Read the model definition and answer for the solid it produces. Units are mm, in the model's axes. Face numbers are marked on the shaded views. A direction names the side the tool comes from. Round coordinates to 2 decimals unless told otherwise and drop trailing zeros. Order: outer loops, then holes, each group sorted by start corner. A loop starts at its lowest first (then second) coordinate and runs counter-clockwise, first axis right, second up. Notation, with made-up numbers: (81.5, 11.25) -> (97.5, 11.25) arc R9 ccw to (97.5, 26.25) -> close; hole circle Ø2 at (59, 86). An arc over 180 degrees is marked (long way). One line per item, written item: value. Start each with the question number.
1. Flat-ended cylindrical pins translate along their axes: pin 1 Ø2.5 at (y, z) = (1.5, -3) entering from +X; pin 2 Ø4 at (x, y) = (34, 6.5) entering from +Z. Find the tip coordinate at first contact, or state that the pin passes through.
2. Section A-A (x = 32) is taken. Give the vertices of the cut face in (y, z), then the cut area to 3 significant figures.
3. The mould has two halves that part along Z. Classify the marked faces 3, 4 and 5: released by +Z, released by -Z, zero draft, split by the parting line, or undercut.
4. Section C-C (z = -2) is taken. Give the vertices of the cut face in (x, y).
5. Section D-D (x = 16.5) is taken. Give the vertices of the cut face in (y, z).
6. For the marked faces 1 and 2, determine the directions among +Z, -Z, +X, -X, +Y, -Y from which every point of the face is accessible in a straight line to the end or side of a thin tool.
7. Consider line 1 (Z direction, x = 25, y = 6); line 2 (X direction, y = 2, z = -2.5); line 3 (X direction, y = 5.75, z = -4.25). Determine where each line is inside the solid, lowest interval first.
8. Section B-B (y = 1.5) is taken. Give the vertices of the cut face in (x, z), then the cut area to 3 significant figures.
from build123d import *

# Parameters (mm, degrees)
SKETCH1_W           = 6.35
SKETCH1_H           = 12.192
BOSS_EXTRUDE1_DEPTH = 25.4
SKETCH2_W           = 1.6002
SKETCH2_H           = 12.192
BOSS_EXTRUDE2_DEPTH = 12.7
CHAMFER1_SIZE       = 10


with BuildPart() as part:
    # Sketch1 → Boss-Extrude1 (new body)
    with BuildSketch(Plane(origin=(0, 0, 0), x_dir=(0, 0, -1), z_dir=(1, 0, 0))):
        with Locations((3.175, 6.096)):
            Rectangle(SKETCH1_W, SKETCH1_H)
    extrude(amount=BOSS_EXTRUDE1_DEPTH)

    # Sketch2 → Boss-Extrude2 (add)
    with BuildSketch(Plane(origin=(25.4, 0, 0), x_dir=(0, 0, -1), z_dir=(1, 0, 0))):
        with Locations((0.8001, 6.096)):
            Rectangle(SKETCH2_W, SKETCH2_H)
        with Locations((5.5499, 6.096)):
            Rectangle(SKETCH2_W, SKETCH2_H)
    extrude(amount=BOSS_EXTRUDE2_DEPTH)

    # Chamfer1
    chamfer1_edges = [part.edges().sort_by_distance(p)[0] for p in [
        (25.4, 12.192, -3.175),
    ]]
    chamfer(chamfer1_edges, length=CHAMFER1_SIZE)


solid = part.part
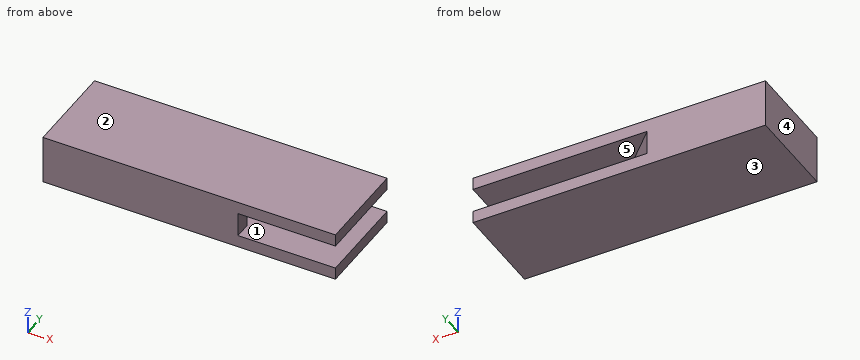
Answer:
1. pin 1: x = 25.4
1. pin 2: z = 0
2. outline: (0, -6.35) -> (12.19, -6.35) -> (12.19, -4.75) -> (0, -4.75) -> close; (0, -1.6) -> (12.19, -1.6) -> (12.19, 0) -> (0, 0) -> close
2. area: 39.0 mm^2
3. face 3: released by -Z
3. face 4: zero draft
3. face 5: undercut
4. outline: (0, 0) -> (25.4, 0) -> (25.4, 2.19) -> (15.4, 12.19) -> (0, 12.19) -> close
5. outline: (0, -6.35) -> (12.19, -6.35) -> (12.19, -4.75) -> (11.09, -4.75) -> (11.09, -1.6) -> (12.19, -1.6) -> (12.19, 0) -> (0, 0) -> close
6. face 1: +X, +Y
6. face 2: +Z, +X, -X, +Y, -Y
7. line 1: -6.35 to -4.75, -1.6 to 0
7. line 2: 0 to 25.4
7. line 3: 0 to 21.84
8. outline: (0, -6.35) -> (38.1, -6.35) -> (38.1, -4.75) -> (25.4, -4.75) -> (25.4, -1.6) -> (38.1, -1.6) -> (38.1, 0) -> (0, 0) -> close
8. area: 202 mm^2
